Verification items for the finished model (mm, model axes). Face numbers are marked on the shaded views. A direction names the side the tool comes from. Coordinates: 2 decimals unless noted, no trailing zeros. Write each loop counter-clockwise with the first axis right and the second up, starting at its lowest first coordinate (ties: lowest second). Pieces come first, ordered by that corner, then holes. Notation, with made-up numbers: (-31, -21) -> (-15, -21) arc R28 ccw to (-15, 18) -> close; hole circle Ø5 at (-38.5, 1.25). An arc over 180 degrees is marked (long way). Write item = value, one per line. Start each with the question number.
(1) Material ranges on probe 1 along X at (y, z) = (6, 4); probe 2 along Y at (x, z) = (11.7, 0); probe 3 along Y at (x, z) = (-0.5, 0), recorded low to high. Write a range as [from, to].
(2) Mould release check, pull along Z, two halves, no side actions. Record for the marked faces 4 and 5: released by +Z, released by -Z, zero draft, split by the parting line, or undercut.
(3) Set-up check for the marked faces 1, 2 and 3: record each of +Z, -Z, +X, -X, +Y, -Y from which the full face is reachable in a straight line by a thin tool's end or side.
(4) Gauge pin test, flat ends, axial feed: pin 1 Ø5 at (x, z) = (-3, -3.5) entering from -Y; pin 2 Ø6 at (x, y) = (-6, -1) entering from -Z; pin 3 Ø1 at (y, z) = (2.5, -1.5) entering from +X; pin 4 Ø4 at (y, z) = (-3, 2) entering from +X. Record the tip position at first contact, or that the pin passes through.
(5) Section check A-A (x = -1.5). Record the cut outline in (y, z).
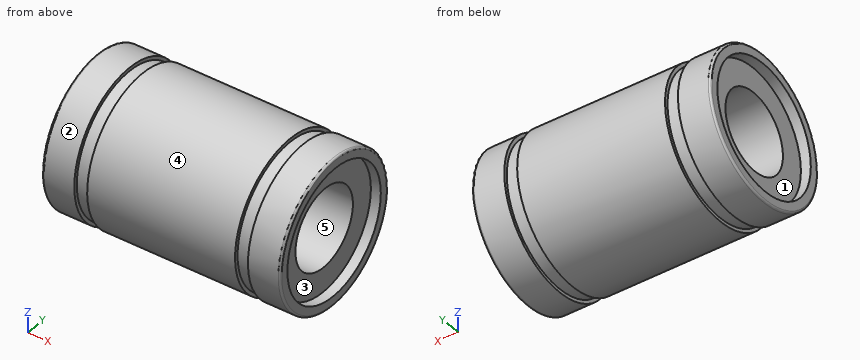
Autodesk Inventor part; units mm, degrees
ref_plane "YZ Plane" through (0, 0, 0) normal (1, 0, 0) x (0, 1, 0)
ref_plane "XZ Plane" through (0, 0, 0) normal (0, 1, 0) x (-1, 0, 0)
ref_plane "XY Plane" through (0, 0, 0) normal (0, 0, 1) x (1, 0, 0)
sketch "Schizzo1" plane through (0, 0, 0) normal (0, 1, 0) x (-1, 0, 0)
  line L0 (-12, 4) -> (-12, 7.5)
  line L1 (-12, 7.5) -> (-8.75, 7.5)
  line L2 (-8.75, 7.5) -> (-8.75, 7.15)
  line L3 (-8.75, 7.15) -> (-7.45, 7.15)
  line L4 (-7.45, 7.15) -> (-7.45, 7.5)
  line L5 (-7.45, 7.5) -> (0, 7.5)
  line L6 (0, 7.5) -> (0, 4)
  line L7 (0, 4) -> (-12, 4)
  line L8 (0, 0) -> (5.7518, 0)
  dimension "d0" = 8
  dimension "d2" = 15
  dimension "d3" = 12
  dimension "d4" = 8.75
  dimension "d5" = 1.3
  dimension "d6" = 14.3
revolve "Rivoluzione1" add sketch "Schizzo1" angle 360 about axis through (0, 0, 0) along (-1, 0, 0)
fillet "Raccordo1" radius 0.2 1 edges at (12, 0, -7.5)
sketch "Schizzo2" plane through (12, 0, 0) normal (1, 0, 0) x (0, 0, -1)
  circle A0 centre (0, 0) radius 7.3
  circle A1 centre (0, 0) radius 6.5
  dimension "d13" = 13
extrude "Estrusione2" cut sketch "Schizzo2" against normal blind 1 contours A1
mirror "Specchio1" about plane through (0, 0, 5.75) normal (-1, 0, 0)
properties part number "LM8UU"
Response:
q1.probe_1 = [-12, -8.75], [-7.45, 7.45], [8.75, 12]
q1.probe_2 = [-7.5, -6.5], [6.5, 7.5]
q1.probe_3 = [-7.5, -4], [4, 7.5]
q2.face_4 = split by the parting line
q2.face_5 = undercut
q3.face_1 = -X
q3.face_2 = +X, -X
q3.face_3 = +X
q4.pin_1 = -7.43
q4.pin_2 = -7.5
q4.pin_3 = through
q4.pin_4 = 11
q5.outline = circle Ø15 at (0, 0); hole circle Ø8 at (0, 0)
